```python
from build123d import *

# Parameters (mm, degrees)
PAD_DEPTH       = 14
FILLET_R        = 5
FILLET001_R     = 3
SKETCH001_R     = 2.25
POCKET_DEPTH    = 9.001
POCKET001_DEPTH = 5


with BuildPart() as part:
    # Sketch → Pad (new body, symmetric)
    with BuildSketch(Plane.XZ):
        with BuildLine():
            Line((-22.5, 0), (0, 0))
            Line((0, 0), (0, 48))
            Line((0, 48), (5, 48))
            Line((5, 48), (5, 10))
            ThreePointArc((5, 10), (7.928932, 2.928932), (15, 0))
            Line((22.5, 0), (15, 0))
            Line((22.5, 0), (22.5, -9))
            Line((22.5, -9), (-22.5, -9))
            Line((-22.5, -9), (-22.5, 0))
        make_face()
    extrude(amount=PAD_DEPTH, both=True)

    # Fillet
    fillet_edges = [part.edges().sort_by_distance(p)[0] for p in [
        (22.5, -14, -4.5),
        (22.5, 14, -4.5),
        (-22.5, -14, -4.5),
        (-22.5, 14, -4.5),
    ]]
    fillet(fillet_edges, radius=FILLET_R)

    # Fillet001
    fillet001_edges = [part.edges().sort_by_distance(p)[0] for p in [
        (0, -14, -9),
        (21.035534, -12.535534, -9),
        (22.5, 0, -9),
        (21.035534, 12.535534, -9),
        (0, 14, -9),
        (-21.035534, 12.535534, -9),
        (-22.5, 0, -9),
        (-21.035534, -12.535534, -9),
        (2.5, -14, 48),
        (2.5, 14, 48),
    ]]
    fillet(fillet001_edges, radius=FILLET001_R)

    # Sketch002 (on DatumPlane) → Groove (revolve, cut)
    with BuildSketch(Plane(origin=(0, 0, 40), x_dir=(0.92388, 0, 0.382683), z_dir=(-0.382683, 0, 0.92388))):
        Polygon((-7, 0), (-7, 0.7), (3, 0.7), (3, 3.8), (5, 3.8), (5, 6), (15, 6), (15, 0), align=None)
    groove = revolve(axis=Axis((0, 0, 40), (0.92388, 0, 0.382683)), mode=Mode.SUBTRACT)

    # Sketch001 → Pocket (cut, through all)
    with BuildSketch(Plane.XY):
        with Locations((-15.75, 0)):
            Circle(SKETCH001_R)
        with Locations((15.75, 0)):
            Circle(SKETCH001_R)
    extrude(amount=-POCKET_DEPTH, mode=Mode.SUBTRACT)

    # Sketch003 → Pocket001 (cut, symmetric)
    with BuildSketch(Plane.XY):
        Polygon((19.35, -2.078461), (19.35, 2.078461), (15.75, 4.156922), (12.15, 2.078461), (12.15, -2.078461), (15.75, -4.156922), align=None)
        Polygon((-12.15, -2.078461), (-12.15, 2.078461), (-15.75, 4.156922), (-19.35, 2.078461), (-19.35, -2.078461), (-15.75, -4.156922), align=None)
    extrude(amount=POCKET001_DEPTH, both=True, mode=Mode.SUBTRACT)

    # Sketch002 LinearPattern 2 → Groove LinearPattern 2 (revolve, cut)
    with BuildSketch(Plane(origin=(0, 12, 40), x_dir=(0.92388, 0, 0.382683), z_dir=(-0.382683, 0, 0.92388))):
        Polygon((-7, 0), (-7, 0.7), (3, 0.7), (3, 3.8), (5, 3.8), (5, 6), (15, 6), (15, 0), align=None)
    groove_linearpattern_2 = revolve(axis=Axis((0, 12, 40), (0.92388, 0, 0.382683)), mode=Mode.SUBTRACT)

    # Mirrored: Groove, Groove LinearPattern 2 across XZ
    add(groove.mirror(Plane.XZ), mode=Mode.SUBTRACT)
    add(groove_linearpattern_2.mirror(Plane.XZ), mode=Mode.SUBTRACT)


solid = part.part
```
Verification items for the finished model (mm, model axes). A direction names the side the tool comes from. Give positions to 0.01 mm unless a question says otherwise; leave off trailing zeros. Order: outer loops, then holes, each group sorted by start corner. A loop starts at its lowest first (then second) coordinate and runs counter-clockwise, first axis right, second up. Notation, with made-up numbers: M -7,54.5 L 42,54.5 A14 cw 42,73.5 Z; hole C 55.25,88 d9. An arc over 180 degrees is marked long. Answer in a Markdown table with one row per item. Add a question column.
Item 1: Mould release check, pull along Z, two halves, no side actions. Record for faces 4 (the flat face through (2, 0, 48)), 5 (the cylindrical face through (3.855, 8.1, 46.532)), 6 (the cylindrical face through (1.508, -0.152, 39.885)), 7 (the flat face through (5, 0, 26)): released by +Z, released by -Z, zero draft, split by the parting line, or undercut.
Item 2: Section check D-D, the plane y = 0. State how many separate pieces and enclosed holes the cut face has, and give its area (3 significant figures).
Item 3: Gauge pin test, flat ends, axial feed: pin 1 (2 mm diameter, centred on y = -10, z = 42, fed in from +X); pin 2 (1 mm diameter, centred on y = -7, z = 21.5, fed in from +X); pin 3 (6 mm diameter, centred on x = 14, y = -0.5, fed in from +Z); pin 4 (3.5 mm diameter, centred on x = 15.75, y = 0, fed in from -Z). Record the tip position at first contact, or that the pin passes through.
Item 4: Scan lines: probe 1 along Y at (x, z) = (-15.75, -6.2); probe 2 along X at (y, z) = (9.25, 25); probe 3 along Z at (x, y) = (-14, 8.25). Record each from-to range of solid material in increasing order. Write a range as from..to.
Item 5: Section check C-C, the plane y = 5. Enter the section's corners in (x, z), and give its area (3 significant figures).
Item 6: Section check A-A, the plane x = -3.5. Enter the section's corners in (y, z), and give its area (3 significant figures).
Item 7: Section check B-B, the plane z = 23. Enter the section's corners in (x, y), and give its area (3 significant figures).
Item 8: Tool access check on faces 1 (the flat face through (-17.58, -3.1, -2.46)), 2 (the flat face through (3.048, 0.084, 45.707)), 3 (the cylindrical face through (1.508, 11.848, 39.885)). Record the directions out of +Z, -Z, +X, -X, +Y, -Y that give a thin tool (end or side, any length) a straight path to the whole face; none if there is none.
Filled sheet:
| question | item | result |
|---|---|---|
| 1 | face 4 | released by +Z |
| 1 | face 5 | undercut |
| 1 | face 6 | undercut |
| 1 | face 7 | zero draft |
| 2 | separate pieces | 4 |
| 2 | enclosed holes | 0 |
| 2 | area | 527 mm^2 |
| 3 | pin 1 | stops at x = 2.83 |
| 3 | pin 2 | stops at x = 5 |
| 3 | pin 3 | stops at z = 0.83 |
| 3 | pin 4 | passes through |
| 4 | probe 1 | y = -13.99..-2.25, 2.25..13.99 |
| 4 | probe 2 | x = 0..5 |
| 4 | probe 3 | z = -9..0 |
| 5 | outline | M -22.5,-6 A3 ccw -19.5,-9 L 19.5,-9 A3 ccw 22.5,-6 L 22.5,0 L 15,0 A10 cw 5,10 L 5,40.99 L 3.35,44.98 L 5,45.66 L 5,48 L 0,48 L 0,0 L -22.5,0 Z |
| 5 | area | 659 mm^2 |
| 6 | outline | M -14,-6 A3 ccw -11,-9 L 11,-9 A3 ccw 14,-6 L 14,0 L -14,0 Z |
| 6 | area | 248 mm^2 |
| 7 | outline | M 0,-14 L 5,-14 L 5,14 L 0,14 Z |
| 7 | area | 140 mm^2 |
| 8 | face 1 | +Z |
| 8 | face 2 | +X |
| 8 | face 3 | none |
